```python
from build123d import *

# Parameters (mm, degrees)
F0_R           = 1.75
F1_DEPTH       = 35
F3_DEPTH       = 11.001
F6_REACH       = 64.9396846637
F8_DEPTH       = 25
F9_R           = 1.25
F10_DEPTH      = 4.2
F12_DEPTH      = 10
F14_DEPTH      = 2
F14_DEPTH_BACK = 2
F16_R          = 1.7
F17_T1_DEPTH   = 30
F17_T4_ANGLE   = 180


# Not quite as in the source:
# - a fillet or chamfer that OpenCascade refuses, or shapes differently, is made with other operations: its cross-section is extruded or revolved along the edge and cut away or added
# - a feature of the source that left no trace in its solid (it failed there, or was rolled back) is left out


with BuildPart() as f1:
    # F0 (on Top) → F1 (new body)
    with BuildSketch(Plane.XY):
        with BuildLine():
            Line((16, 5.5), (-16, 5.5))
            ThreePointArc((-16, 5.5), (-21.5, 0), (-16, -5.5))
            Line((-16, -5.5), (16, -5.5))
            ThreePointArc((16, -5.5), (21.5, 0), (16, 5.5))
        make_face()
        with Locations((-16, 0)):
            Circle(F0_R, mode=Mode.SUBTRACT)
        with Locations((16, 0)):
            Circle(F0_R, mode=Mode.SUBTRACT)
    extrude(amount=F1_DEPTH)

    # F2 (on face) → F3 (cut, through all)
    with BuildSketch(Plane.XZ.offset(5.5)):
        with BuildLine():
            Line((-8.5, 35), (-8.5, 17.5))
            ThreePointArc((-8.5, 17.5), (0, 9), (8.5, 17.5))
            Line((8.5, 17.5), (8.5, 35))
            Line((8.5, 35), (-8.5, 35))
        make_face()
    extrude(amount=-F3_DEPTH, mode=Mode.SUBTRACT)

    f6_end = Plane(origin=(0, -5.5, 14.4059555713), x_dir=(0, 0, -1), z_dir=(0, -1, 0))
    # F5 (on face) → F6 (join, up to a plane its end follows)
    with BuildSketch(Plane(origin=(0, -5.1315698604, -1.375), x_dir=(-1, 0, 0), z_dir=(0, 0.9659258263, 0.2588190451))):
        with BuildLine():
            ThreePointArc((16, 32.3272067081), (15.4142135624, 33.7414202705), (14, 34.3272067081))
            Line((14, 34.3272067081), (-14, 34.3272067081))
            ThreePointArc((-14, 34.3272067081), (-15.4142135624, 33.7414202705), (-16, 32.3272067081))
            Line((-16, 32.3272067081), (-16, 4.3272067081))
            ThreePointArc((-16, 4.3272067081), (-15.4142135624, 2.9129931457), (-14, 2.3272067081))
            Line((-14, 2.3272067081), (14, 2.3272067081))
            ThreePointArc((14, 2.3272067081), (15.4142135624, 2.9129931457), (16, 4.3272067081))
            Line((16, 4.3272067081), (16, 32.3272067081))
        make_face()
    f6_long = extrude(amount=F6_REACH, mode=Mode.PRIVATE)
    add(split(f6_long, bisect_by=f6_end, keep=Keep.TOP, mode=Mode.PRIVATE))

    # F7 (on face) → F8 (cut)
    with BuildSketch(Plane(origin=(0, 5.5, 0), x_dir=(-1, 0, 0), z_dir=(0, 1, 0))):
        with BuildLine():
            Line((8.5, 35), (-8.5, 35))
            Line((-8.5, 35), (-8.5, 17.5))
            ThreePointArc((-8.5, 17.5), (0, 9), (8.5, 17.5))
            Line((8.5, 17.5), (8.5, 35))
        make_face()
    extrude(amount=-F8_DEPTH, mode=Mode.SUBTRACT)

    # F9 (on face) → F10 (cut)
    with BuildSketch(Plane(origin=(0, -5.1315698604, -1.375), x_dir=(1, 0, 0), z_dir=(0, -0.9659258263, -0.2588190451))):
        with Locations((-14, 32.3272067081)):
            Circle(F9_R)
        with Locations((14, 32.3272067081)):
            Circle(F9_R)
        with Locations((14, 4.3272067081)):
            Circle(F9_R)
        with Locations((-14, 4.3272067081)):
            Circle(F9_R)
    extrude(amount=-F10_DEPTH, mode=Mode.SUBTRACT)

    # F11 (on face) → F12 (cut)
    with BuildSketch(Plane(origin=(0, -5.1315698604, -1.375), x_dir=(1, 0, 0), z_dir=(0, -0.9659258263, -0.2588190451))):
        with BuildLine():
            Line((8.5, 19.5408379052), (8.5, 26.8272067081))
            Line((8.5, 26.8272067081), (-8.5, 26.8272067081))
            Line((-8.5, 26.8272067081), (-8.5, 19.5408379052))
            add(Edge.make_bspline(
                [(8.5, 19.5408379052), (8.5, 10.7409903718), (0, 10.7409903718), (-8.5, 10.7409903718), (-8.5, 19.5408379052)],
                knots=[4.7123889804, 4.7123889804, 4.7123889804, 6.2831853072, 6.2831853072, 7.853981634, 7.853981634, 7.853981634], degree=2, weights=[1, 0.7071067812, 1, 0.7071067812, 1]))
        make_face()
        with BuildLine():
            Line((12, 9.8272067081), (12, 26.8272067081))
            Line((12, 26.8272067081), (8.5, 26.8272067081))
            Line((8.5, 26.8272067081), (8.5, 19.5408379052))
            add(Edge.make_bspline(
                [(8.5, 19.5408379052), (8.5, 10.7409903718), (0, 10.7409903718), (-8.5, 10.7409903718), (-8.5, 19.5408379052)],
                knots=[4.7123889804, 4.7123889804, 4.7123889804, 6.2831853072, 6.2831853072, 7.853981634, 7.853981634, 7.853981634], degree=2, weights=[1, 0.7071067812, 1, 0.7071067812, 1]))
            Line((-8.5, 19.5408379052), (-8.5, 26.8272067081))
            Line((-8.5, 26.8272067081), (-12, 26.8272067081))
            Line((-12, 26.8272067081), (-12, 9.8272067081))
            Line((-12, 9.8272067081), (12, 9.8272067081))
        make_face()
    extrude(amount=-F12_DEPTH, mode=Mode.SUBTRACT)

    # F13 (on face) → F14 (join, two sides)
    with BuildSketch(Plane.YZ.offset(16)) as f14_sk:
        with BuildLine():
            ThreePointArc((5.5, 0), (16.3836762358, 17.5), (5.5, 35))
            Line((5.5, 35), (5.5, 0))
        make_face()
    extrude(amount=F14_DEPTH)
    extrude(f14_sk.sketch, amount=-F14_DEPTH_BACK)

    # F15: F1 across plane


with BuildPart() as f1_1:
    add(f1.part)
    add(f1.part.mirror(Plane.YZ))

    # F16
    f16_edges = [f1_1.edges().sort_by_distance(p)[0] for p in [
        (18, 16.383676, 17.5),
        (14, 16.383676, 17.5),
        (-14, 16.383676, 17.5),
        (-18, 16.383676, 17.5),
    ]]
    fillet(f16_edges, radius=F16_R)

    # F17: fillet of radius 5 on 3 edges, made by hand

    # F17_s2 → F17_t1 (cut)
    with BuildSketch(Plane.XY.offset(17.5)):
        with BuildLine():
            ThreePointArc((13.5, 5.5), (9.9644660941, 4.0355339059), (8.5, 0.5))
            Line((8.5, 0.5), (8.5, 5.5))
            Line((8.5, 5.5), (13.5, 5.5))
        make_face()
        with BuildLine():
            ThreePointArc((-13.5, 5.5), (-9.9644660941, 4.0355339059), (-8.5, 0.5))
            Line((-8.5, 0.5), (-8.5, 5.5))
            Line((-8.5, 5.5), (-13.5, 5.5))
        make_face()
    extrude(amount=F17_T1_DEPTH, mode=Mode.SUBTRACT)

    # F17_s3 → F17_t4 (revolve, cut)
    with BuildSketch(Plane.XY.offset(17.5)):
        with BuildLine():
            ThreePointArc((-13.5, 5.5), (-9.9644660941, 4.0355339059), (-8.5, 0.5))
            Line((-8.5, 0.5), (-8.5, 5.5))
            Line((-8.5, 5.5), (-13.5, 5.5))
        make_face()
    revolve(axis=Axis((0, 5.5, 17.5), (0, -1, 0)), revolution_arc=F17_T4_ANGLE, mode=Mode.SUBTRACT)


solid = f1_1.part
```
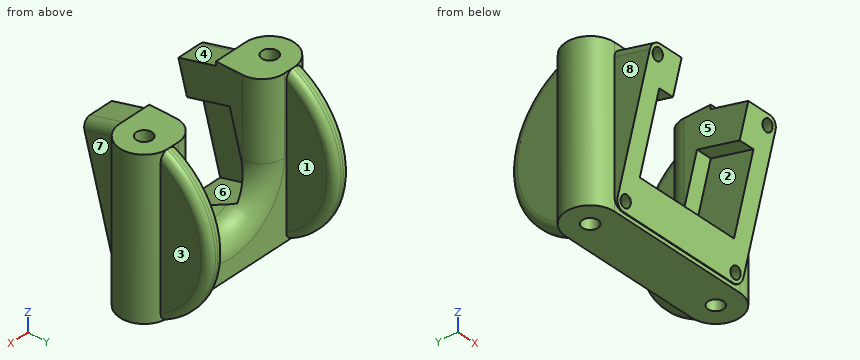
Verification items for the finished model (mm, model axes). Face numbers are marked on the shaded views. A direction names the side the tool comes from. Coordinates: 2 decimals unless noted, no trailing zeros. Loops run counter-clockwise (first coordinate to the right, second up) from the corner with the lowest first, then second, coordinate; pieces in that order, holes last. Notation, with made-up numbers: (73.5, 78.5) -> (121.5, 78.5) arc R20 cw to (121.5, 114.5) -> close; hole circle Ø7 at (67.25, 46.5). An arc over 180 degrees is marked (long way). Answer in a Markdown table with one row per item.
1) Depth check by flat-ended pin: P1, Ø7.5, axis at y = 8.5, z = 16.5, coming from the -X side; P2, Ø3, axis at y = 12, z = 19, coming from the +X side; P3, Ø4, axis at y = -8, z = 23, coming from the -X side; P4, Ø3, axis at x = -16, y = 0, coming from the -Z side (3 decimals). Enter the tip coordinate at first touch or a pass-through.
The answers:
| item | result |
|---|---|
| P1 | stops at x = -18.77 |
| P2 | stops at x = 18 |
| P3 | stops at x = -16 |
| P4 | passes through |
2) Section check A-A (x = 17). Record the cut outline in (y, z), and give its area (3 significant figures).
The answers:
| item | result |
|---|---|
| outline | (-5.41, 0) -> (-1.44, 0) -> (-1.44, 35) -> (-5.41, 35) -> close; (1.44, 0) -> (5.41, 0) -> (5.41, 35) -> (1.44, 35) -> close; (5.5, 0.17) arc R19.36 ccw to (5.5, 34.83) -> close |
| area | 544 mm2 |
3) Section check B-B (z = 21). Give the number of separate pieces and of enclosed holes in the cut face, and give its area (3 significant figures).
The answers:
| item | result |
|---|---|
| separate pieces | 2 |
| enclosed holes | 2 |
| area | 324 mm2 |
4) Access from +Z, -Z, +X, -X, +Y, -Y to the whole of each face (thin tool, end or side, straight path). Record for the marked faces 5, 6, 7 and 8.
The answers:
| item | result |
|---|---|
| face 5 | +Z, +Y, -Y |
| face 6 | -Y |
| face 7 | +Z, -Z, +X, -Y |
| face 8 | +Z, -Z, -X, -Y |
5) Draft check along X on the marked faces 1, 2, 3 and 4. Enter one of: released by +X, released by -X, zero draft, split by the parting line, or undercut.
The answers:
| item | result |
|---|---|
| face 1 | undercut |
| face 2 | undercut |
| face 3 | released by +X |
| face 4 | zero draft |
6) Scan lines: line 1 along X through (y, z) = (-8, 13); line 2 along X through (y, z) = (6.5, 10); line 3 along X through (y, z) = (1, 29). Record each from-to range of solid material in increasing order. Write a range as from..to.
The answers:
| item | result |
|---|---|
| line 1 | x = -16..-12, 12..16 |
| line 2 | x = -18..-14, 14..18 |
| line 3 | x = -21.41..-17.44, -14.56..-8.53, 8.53..14.56, 17.44..21.41 |
